Autodesk Inventor part; units mm, degrees
ref_plane "YZ Plane" through (0, 0, 0) normal (1, 0, 0) x (0, 1, 0)
ref_plane "XZ Plane" through (0, 0, 0) normal (0, 1, 0) x (-1, 0, 0)
ref_plane "XY Plane" through (0, 0, 0) normal (0, 0, 1) x (1, 0, 0)
sketch "Sketch1" plane through (0, 0, 0) normal (0, 0, 1) x (1, 0, 0)
  line L0 (-13, 12) -> (13, 12)
  line L1 (13, 12) -> (13, -12)
  line L2 (13, -12) -> (-13, -12)
  line L3 (-13, -12) -> (-13, 12)
  line L4 (-13, 3.25) -> (-15, 3.25)
  line L5 (-15, 3.25) -> (-15, -3.25)
  line L6 (-15, -3.25) -> (-13, -3.25)
  line L7 (-13, -3.25) -> (-13, 3.25)
  line L8 (13, 3.25) -> (15, 3.25)
  line L9 (15, 3.25) -> (15, -3.25)
  line L10 (15, -3.25) -> (13, -3.25)
  line L11 (13, -3.25) -> (13, 3.25)
  line L12 (-25.4, 25.4) -> (25.4, 25.4)
  line L13 (25.4, 25.4) -> (25.4, -25.4)
  line L14 (25.4, -25.4) -> (-25.4, -25.4)
  line L15 (-25.4, -25.4) -> (-25.4, 25.4)
  circle A0 centre (0, 0) radius 7.1437
  circle A1 centre (-3, 12) radius 1.5
  line L16 (-13, 8) -> (-9, 12)
  line L17 (9, 12) -> (13, 8)
  line L18 (13, -8) -> (9, -12)
  line L19 (-13, -8) -> (-9, -12)
  circle A2 centre (0, 0) radius 20.8915
  circle A3 centre (-21.997, 0) radius 1.5875
  circle A4 centre (10.9985, 19.05) radius 1.5875
  circle A5 centre (10.9985, -19.05) radius 1.5875
  circle A6 centre (0, 0) radius 21.997 construction
  point P0 (-14, 3.25)
  point P1 (14, 3.25)
  point P2 (-14, -3.25)
  point P3 (14, -3.25)
  point P4 (-20.32, 20.32)
  point P5 (20.32, 20.32)
  point P6 (20.32, -20.32)
  point P7 (-20.32, -20.32)
  dimension "d0" = 24
  dimension "d1" = 12
  dimension "d2" = 26
  dimension "d3" = 13
  dimension "d4" = 2
  dimension "d5" = 6.5
  dimension "d6" = 3.25
  dimension "d7" = 2
  dimension "d8" = 14.2875
  dimension "d9" = 50.8
  dimension "d10" = 25.4
  dimension "d11" = 50.8
  dimension "d12" = 25.4
  dimension "d13" = 3
  dimension "d14" = 10
  dimension "d15" = 4
  dimension "d16" = 4
  dimension "d17" = 4
  dimension "d18" = 4
  dimension "d19" = 4
  dimension "d20" = 5.08
  dimension "d21" = 5.08
  dimension "d22" = 5.08
  dimension "d23" = 5.08
  dimension "d34" = 40.64
  dimension "d35" = 40.64
  dimension "d44" = 41.783
  dimension "d45" = 3.175
  dimension "d46" = 3.175
  dimension "d47" = 3.175
  dimension "d48" = 38.1
  dimension "d49" = 38.1
  dimension "d50" = 38.1
  dimension "d51" = 38.1
  dimension "d53" = 43.9941
extrude "Extrusion1" add sketch "Sketch1" against normal blind 3.175 contours L0 L16 L3 | L0 L1 L17 | L19 L2 L3 | L18 L1 L2 | L12 L13 L14 L15 | A2 A5 A3 A4 | A4 A2 | A2 A4 | A5 A2 | A2 A5 | A3 A2 | A2 A3
fillet "Fillet1" radius 3.175 4 edges at (-13, -3.25, -1.5875) (-13, 3.25, -1.5875) (13, 3.25, -1.5875) (13, -3.25, -1.5875)
hole "Hole1" at (-20.32, 20.32, 0) at (20.32, 20.32, 0) at (20.32, -20.32, 0) at (-20.32, -20.32, 0) direction (0, 0, -1) diameter 4.572 end through all
extrude "Extrusion2" cut sketch "Sketch1" against normal blind 25.4 contours L0 L16 L3 | L0 A1 L17 L1 L18 L2 L19 L3 L16 | L0 A1 | L0 L1 L17 | L19 L2 L3 | L18 L1 L2 | A0 | A2 A5 A3 A4 | A4 A2 | A2 A5 | A3 A2 picked at (-3.284, 11.1238) picked at (10.4165, 17.9252) picked at (10.4165, -17.9252) picked at (-20.7286, 0)
fillet "Fillet2" radius 6.35 4 edges at (25.4, 25.4, -1.5875) (-25.4, 25.4, -1.5875) (25.4, -25.4, -1.5875) (-25.4, -25.4, -1.5875)
equation "\"d7\" = d4"
equation "\"d16\" = d15"
equation "\"d17\" = d15"
equation "\"d18\" = d15"
equation "\"d19\" = d15"
equation "\"d46\" = d45"
equation "\"d47\" = d45"
properties part number "BD gearbox mount block"
Check sheet for the modelled part. Datum: model origin and axes. Units: mm. Round coordinates to 2 decimals unless told otherwise and drop trailing zeros. Loops run counter-clockwise (first coordinate to the right, second up) from the corner with the lowest first, then second, coordinate; pieces in that order, holes last. Notation, with made-up numbers: (41, 52) -> (92, 52) arc R32 cw to (92, 82) -> close; hole circle Ø1 at (4.25, 77). An arc over 180 degrees is marked (long way). Put each result on its own line as item: value. Start each with the question number.
1. Draft check along X on faces 1 (the face through (18.775, 22.005, -1.61)), 2 (the face through (-23.59, 23.49, -1.61)), 3 (the face through (18.392, -21.549, -1.61)), 4 (the face through (22, 0, 0)). Enter one of: +X half, -X half, draft (parallel to the pull), parting line (faces both ways), or undercut.
2. Scan lines: probe 1 along Y at (x, z) = (-22, -1.8); probe 2 along X at (y, z) = (-19, -2.35); probe 3 along X at (y, z) = (-18, -0.55). Record each from-to range of solid material in increasing order.
3. Section check C-C (z = -0.6). Enter the section's corners in (x, y), plus the area to 3 significant figures.
4. Section check B-B (y = -11). Enter the section's corners in (x, z) (3 decimals), plus the area to 3 significant figures.
5. Section check A-A (x = 0). Enter the section's corners in (y, z) (1 decimal).
6. Gauge pin test, flat end, axial feed: pin 1 (5.5 mm diameter, centred on x = 20.32, y = 20.32, fed in from -Z) (3 decimals). Record the tip position at first contact, or that the pin passes through.
Findings:
1. face 1: undercut
1. face 2: -X half
1. face 3: undercut
1. face 4: draft
2. probe 1: y = -24.67 to -21.87, -18.77 to 18.77, 21.87 to 24.67
2. probe 2: x = -25.4 to -22.19, -18.45 to -8.69, 8.69 to 18.45, 22.19 to 25.4
2. probe 3: x = -25.4 to -10.6, 10.6 to 25.4
3. outline: (-25.4, -19.05) arc R6.35 ccw to (-19.05, -25.4) -> (19.05, -25.4) arc R6.35 ccw to (25.4, -19.05) -> (25.4, 19.05) arc R6.35 ccw to (19.05, 25.4) -> (-19.05, 25.4) arc R6.35 ccw to (-25.4, 19.05) -> close; hole circle Ø4.57 at (-20.32, -20.32); hole circle Ø4.57 at (-20.32, 20.32); hole circle Ø41.78 at (0, 0); hole circle Ø4.57 at (20.32, -20.32); hole circle Ø4.57 at (20.32, 20.32)
3. area: 1,110 mm^2
4. outline: (-25.4, -3.175) -> (-17.761, -3.175) -> (-17.761, 0) -> (-25.4, 0) -> close; (17.761, -3.175) -> (25.4, -3.175) -> (25.4, 0) -> (17.761, 0) -> close
4. area: 48.5 mm^2
5. outline: (-25.4, -3.2) -> (-20.9, -3.2) -> (-20.9, 0) -> (-25.4, 0) -> close; (20.9, -3.2) -> (25.4, -3.2) -> (25.4, 0) -> (20.9, 0) -> close
6. pin 1: stops at z = -3.175
